Model file for the job. Use its own axes, mm. A direction names the side the tool comes from. Round coordinates to 2 decimals unless told otherwise and drop trailing zeros. Order: outer loops, then holes, each group sorted by start corner. A loop starts at its lowest first (then second) coordinate and runs counter-clockwise, first axis right, second up. Notation, with made-up numbers: (33.5, 39.25) - (85.5, 39.25) arc R12 ccw to (85.5, 60.25) - close; hole circle Ø3 at (55, 37). An arc over 180 degrees is marked (long way). Answer as CSV lines item,"result". Start each with the question number.
1. Pin check, flat tips, straight feed: pin 1 Ø4.5 at (x, y) = (-45.5, 12) entering from +Z; pin 2 Ø10 at (y, z) = (8, -15.5) entering from +X; pin 3 Ø8 at (y, z) = (17, -30) entering from +X; pin 4 Ø3 at (x, z) = (-47, -7.5) entering from -Y. Stop position of each tip, or through.
2. Band-saw the part on D-D on z = -6.5. List the corners of the cut face in (x, y).
3. Wall check: line 1 along X through (y, z) = (11, -34); line 2 along Y through (x, z) = (-27.5, -30); line 3 along X through (y, z) = (2.75, -35). Give the ranges that are in metal, low to high. Write a range as [from, to].
4. 3-axis set-ups, long thin cutter, end or side, ignore diameter. For faces 4 (the face through (-25, 11.5, -29.9)), 5 (the face through (-40, 7, -30)), 6 (the face through (-40, 6, -20)), 7 (the face through (-41, 2, -16)): which of +Z, -Z, +X, -X, +Y, -Y reach the whole face in a straight line?
5. Pull direction X, two halves, no side cores. Call faces 1 (the face through (-10, 1, -25)), 2 (the face through (-45, 15, -25)), 3 (the face through (-40, 6, -40)): released by +X, released by -X, zero draft, split by the parting line, or undercut.
6. Band-saw the part on B-B on z = -33. List the corners of the cut face in (x, y).
7. Band-saw the part on C-C on y = 19.75. List the corners of the cut face in (x, z), then the cut area to 3 significant figures.
```python
from build123d import *

# Parameters (mm, degrees)
SKETCH1_W           = 80
SKETCH1_H           = 40
BOSS_EXTRUDE1_DEPTH = 2
CUT_EXTRUDE1_DEPTH  = 5
SKETCH3_W           = 30
SKETCH3_H           = 20
BOSS_EXTRUDE2_DEPTH = 25
SKETCH4_R           = 5
CUT_EXTRUDE2_DEPTH  = 74.17103252
SKETCH5_W           = 10
SKETCH5_H           = 20
CUT_EXTRUDE3_DEPTH  = 20
FILLET1_R           = 10


with BuildPart() as part:
    # Sketch1 → Boss-Extrude1 (new body)
    with BuildSketch(Plane(origin=(0, 0, 0), x_dir=(1, 0, 0), z_dir=(0, 1, 0))):
        with Locations((-40, 20)):
            Rectangle(SKETCH1_W, SKETCH1_H)
    extrude(amount=BOSS_EXTRUDE1_DEPTH)

    # Sketch2 → Cut-Extrude1 (cut)
    with BuildSketch(Plane(origin=(0, 2, 0), x_dir=(1, 0, 0), z_dir=(0, 1, 0))):
        Polygon((-80, 10), (-60, 40), (-80, 40), align=None)
        Polygon((0, 10), (-20, 40), (0, 40), align=None)
    extrude(amount=-CUT_EXTRUDE1_DEPTH, mode=Mode.SUBTRACT)

    # Sketch3 → Boss-Extrude2 (add)
    with BuildSketch(Plane(origin=(0, 2, 0), x_dir=(1, 0, 0), z_dir=(0, 1, 0))):
        with Locations((-40, 30)):
            Rectangle(SKETCH3_W, SKETCH3_H)
    extrude(amount=BOSS_EXTRUDE2_DEPTH)

    # Sketch4 → Cut-Extrude2 (cut, through all)
    with BuildSketch(Plane(origin=(-25, 0, 0), x_dir=(0, 0, -1), z_dir=(1, 0, 0))):
        with Locations((30, 17)):
            Circle(SKETCH4_R)
    extrude(amount=-CUT_EXTRUDE2_DEPTH, mode=Mode.SUBTRACT)

    # Sketch5 → Cut-Extrude3 (cut)
    with BuildSketch(Plane(origin=(0, 27, 0), x_dir=(1, 0, 0), z_dir=(0, 1, 0))):
        with Locations((-40, 30)):
            Rectangle(SKETCH5_W, SKETCH5_H)
    extrude(amount=-CUT_EXTRUDE3_DEPTH, mode=Mode.SUBTRACT)

    # Fillet1
    fillet1_edges = [part.edges().sort_by_distance(p)[0] for p in [
        (-30, 27, -20),
        (-50, 27, -20),
        (-50, 27, -40),
        (-30, 27, -40),
    ]]
    fillet(fillet1_edges, radius=FILLET1_R - 0.0001)  # a hair under: the kernel refuses the full size


solid = part.part
```
Reply:
1,pin 1,"stops at z = -20"
1,pin 2,"stops at x = -25"
1,pin 3,"passes through"
1,pin 4,"stops at y = 0"
2,outline,"(-80, 0) - (0, 0) - (0, 2) - (-80, 2) - close"
3,line 1,"x = [-55, -45], [-35, -25]"
3,line 2,"y = [0, 12], [22, 27]"
3,line 3,"x = [-55, -25]"
4,face 4,"+Z, -Z, +X, +Y"
4,face 5,"+Z, -Z, +Y"
4,face 6,"+Z, +X, -X, +Y"
4,face 7,"+Z, +Y"
5,face 1,"released by +X"
5,face 2,"undercut"
5,face 3,"zero draft"
6,outline,"(-64.67, 0) - (-15.33, 0) - (-15.33, 2) - (-25, 2) - (-25, 13) - (-35, 13) - (-35, 7) - (-45, 7) - (-45, 13) - (-55, 13) - (-55, 2) - (-64.67, 2) - close; (-55, 21) - (-45, 21) - (-45, 26.54) - (-55, 26.54) - close; (-35, 21) - (-25, 21) - (-25, 26.54) - (-35, 26.54) - close"
7,outline,"(-55, -39.61) - (-45, -39.61) - (-45, -34.18) - (-55, -34.18) - close; (-55, -25.82) - (-45, -25.82) - (-45, -20.39) - (-55, -20.39) - close; (-35, -39.61) - (-25, -39.61) - (-25, -34.18) - (-35, -34.18) - close; (-35, -25.82) - (-25, -25.82) - (-25, -20.39) - (-35, -20.39) - close"
7,area,"218 mm2"
